from build123d import *

# Parameters (mm, degrees)
BOSS_EXTRUDE1_DEPTH = 100


with BuildPart() as part:
    # Sketch1 → Boss-Extrude1 (new body)
    with BuildSketch(Plane(origin=(0, 0, 0), x_dir=(1, 0, 0), z_dir=(0, 1, 0))):
        Polygon((2.0975, 3.632976569), (-2.0975, 3.632976569), (-4.195, 0), (-2.0975, -3.632976569), (2.0975, -3.632976569), (4.195, 0), align=None)
    extrude(amount=-BOSS_EXTRUDE1_DEPTH)


solid = part.part
For this review, take the finished solid that the model builds, in its own axes (mm). Round coordinates to 2 decimals unless told otherwise and drop trailing zeros. Order: outer loops, then holes, each group sorted by start corner. A loop starts at its lowest first (then second) coordinate and runs counter-clockwise, first axis right, second up. Notation, with made-up numbers: M -31,5 L 24,5 A22 cw 24,44 Z; hole C -23,13.25 d11. An arc over 180 degrees is marked long. Use a Markdown table: item, result. Add a question column.
Item 1: Add section A-A, the plane y = -29.5. Give the boundary of the cut face in (x, z) (1 decimal), then the cut area to 3 significant figures.
Item 2: Add section B-B, the plane z = 1. Give the boundary of the cut face in (x, y), then the cut area to 3 significant figures.
Item 3: Insertion check: pin 1 (3 mm diameter, centred on x = -1.5, z = -0.5, fed in from +Y); pin 2 (1 mm diameter, centred on y = -10.5, z = -1, fed in from -X). Each pin has a flat end and moves straight along its axis. Give the tip position at first contact, or say it passes through.
Item 4: Mouldability with a two-part tool opening along Z and no side actions: class faces 1 (the flat face through (0, -100, 0)), 2 (the flat face through (0, -49, -3.633)), 3 (the flat face through (0, -49, 3.633)) as released by +Z, released by -Z, zero draft, split by the parting line, or undercut.
Item 5: To check wall thickness, follow line 1 along Z through (x, y) = (2.5, -8.5); line 2 along X through (y, z) = (-30, -1.25); line 3 along X through (y, z) = (-85, 2.5). State the ranges of each line that lie inside material, in increasing order.
Geometry results:
| question | item | result |
|---|---|---|
| 1 | outline | M -4.2,0 L -2.1,-3.6 L 2.1,-3.6 L 4.2,0 L 2.1,3.6 L -2.1,3.6 Z |
| 1 | area | 45.7 mm² |
| 2 | outline | M -3.62,-100 L 3.62,-100 L 3.62,0 L -3.62,0 Z |
| 2 | area | 724 mm² |
| 3 | pin 1 | stops at y = 0 |
| 3 | pin 2 | stops at x = -3.91 |
| 4 | face 1 | zero draft |
| 4 | face 2 | released by -Z |
| 4 | face 3 | released by +Z |
| 5 | line 1 | z = -2.94 to 2.94 |
| 5 | line 2 | x = -3.47 to 3.47 |
| 5 | line 3 | x = -2.75 to 2.75 |
